```python
from build123d import *

# Parameters (mm, degrees)
SZKIC1_W                    = 140
SZKIC1_H                    = 50
DODANIE_WYCI_GNI_CIE1_DEPTH = 2
DODANIE_WYCI_GNI_CIE2_DEPTH = 12
SFAZOWANIE1_SIZE            = 5


with BuildPart() as part:
    # Szkic1 → Dodanie-wyciągnięcie1 (new body)
    with BuildSketch(Plane.XY):
        Rectangle(SZKIC1_W, SZKIC1_H)
        with BuildLine():
            ThreePointArc((-14.432240892, 12.367994391), (-11.873973335, 6.417701356), (-11, 0))
            ThreePointArc((-11, 0), (-13.243691419, -10.132276987), (-19.555253078, -18.370078729))
            ThreePointArc((-19.555253078, -18.370078729), (-18.936918944, -19.082957273), (-18.714285714, -20))
            ThreePointArc((-18.714285714, -20), (-20.427440625, -21.97932309), (-22.632005609, -20.567759108))
            ThreePointArc((-22.632005609, -20.567759108), (-38.945575695, -23.673454172), (-53.370078729, -15.444746922))
            ThreePointArc((-53.370078729, -15.444746922), (-56.627466942, -15.448190673), (-55.567759108, -12.367994391))
            ThreePointArc((-55.567759108, -12.367994391), (-58.673454172, 3.945575695), (-50.444746922, 18.370078729))
            ThreePointArc((-50.444746922, 18.370078729), (-50.448190673, 21.627466942), (-47.367994391, 20.567759108))
            ThreePointArc((-47.367994391, 20.567759108), (-31.054424305, 23.673454172), (-16.629921271, 15.444746922))
            ThreePointArc((-16.629921271, 15.444746922), (-14.391659035, 16.190949513), (-13, 14.285714286))
            ThreePointArc((-13, 14.285714286), (-13.397577113, 13.088951614), (-14.432240892, 12.367994391))
        make_face(mode=Mode.SUBTRACT)
        with BuildLine():
            ThreePointArc((50.444746922, 18.370078729), (56.756308581, 10.132276987), (59, 0))
            ThreePointArc((59, 0), (58.126026665, -6.417701356), (55.567759108, -12.367994391))
            ThreePointArc((55.567759108, -12.367994391), (56.602422887, -13.088951614), (57, -14.285714286))
            ThreePointArc((57, -14.285714286), (55.608340965, -16.190949513), (53.370078729, -15.444746922))
            ThreePointArc((53.370078729, -15.444746922), (38.945575695, -23.673454172), (22.632005609, -20.567759108))
            ThreePointArc((22.632005609, -20.567759108), (19.551809327, -21.627466942), (19.555253078, -18.370078729))
            ThreePointArc((19.555253078, -18.370078729), (11.326545828, -3.945575695), (14.432240892, 12.367994391))
            ThreePointArc((14.432240892, 12.367994391), (13.372533058, 15.448190673), (16.629921271, 15.444746922))
            ThreePointArc((16.629921271, 15.444746922), (31.054424305, 23.673454172), (47.367994391, 20.567759108))
            ThreePointArc((47.367994391, 20.567759108), (49.572559375, 21.97932309), (51.285714286, 20))
            ThreePointArc((51.285714286, 20), (51.063081056, 19.082957273), (50.444746922, 18.370078729))
        make_face(mode=Mode.SUBTRACT)
    extrude(amount=DODANIE_WYCI_GNI_CIE1_DEPTH)

    # Szkic2 → Dodanie-wyciągnięcie2 (add)
    with BuildSketch(Plane.XY.offset(2)):
        Polygon((70, 25), (70, -19), (82, -19), (82, -13), (72, -13), (72, 27), (-72, 27), (-72, -13), (-82, -13), (-82, -19), (-70, -19), (-70, 25), align=None)
    extrude(amount=-DODANIE_WYCI_GNI_CIE2_DEPTH)

    # Szkic4 → CBORE for M3 Hex Socket Head Cap Screw1 (revolve, cut)
    with BuildSketch(Plane(origin=(-77, -13, -4), x_dir=(0, 0, 1), z_dir=(1, 0, 0))):
        Polygon((0, 0), (0, 8.66137699), (1.6, 7.7), (1.6, 3.4), (3.25, 3.4), (3.25, 0), align=None)
    cbore_for_m3_hex_socket_head_cap_screw1 = revolve(axis=Axis((-77, -6.65, -4), (0, -1, 0)), mode=Mode.SUBTRACT)

    # Lustro1: CBORE for M3 Hex Socket Head Cap Screw1 across plane
    add(cbore_for_m3_hex_socket_head_cap_screw1.mirror(Plane(origin=(0, 0, 0), x_dir=(0, 0, 1), z_dir=(1, 0, 0))), mode=Mode.SUBTRACT)

    # Sfazowanie1
    # the kernel refuses this chamfer: 5 mm, written as the material it takes off along each edge
    with BuildSketch(Plane(origin=(-82, -13, 14.85841494), x_dir=(0.9996219169112968, 0.027495876610586625, 0), z_dir=(0, 0, -1)), Plane(origin=(82, -13, 14.85841494), x_dir=(0.027495876610590466, -0.9996219169112965, 0), z_dir=(0, 0, -1))) as sfazowanie1_piece_1:
        Polygon((SFAZOWANIE1_SIZE * 0.999621916911, SFAZOWANIE1_SIZE * 0.0274958766106), (-SFAZOWANIE1_SIZE * 0.0274958766106, SFAZOWANIE1_SIZE * 0.999621916911), (0, 0), align=None)
    extrude(amount=37.71682988, mode=Mode.SUBTRACT)


solid = part.part
```
CAD build for the part. Positions are in the model's coordinates, mm. A direction names the side the tool comes from. Give positions to 0.01 mm unless a question says otherwise; leave off trailing zeros. Order: outer loops, then holes, each group sorted by start corner. A loop starts at its lowest first (then second) coordinate and runs counter-clockwise, first axis right, second up.
(1) Drill centre lines: L1, parallel to X at y = -18.2, z = -4; L2, parallel to X at y = 8.5, z = 1; L3, parallel to X at y = 13.5, z = 0.5. Where is each one in solid material? Low to high.
(2) Flat gauge pins, fed straight in: pin 1 (2.5 mm diameter, centred on x = 20.71, y = -20, fed in from -Z); pin 2 (4.5 mm diameter, centred on x = -55, y = -14.29, fed in from -Z); pin 3 (3 mm diameter, centred on x = 28, z = -5, fed in from -Y); pin 4 (1 mm diameter, centred on y = -21, z = 1, fed in from +X). Where does each tip first touch, or does it go through?
(3) Saw through at C-C, the plane x = -1. Give the cut face in (y, z).
(4) Mould opens along Z. For faces 1 (the flat face through (75, -19, -4)), 2 (the cylindrical face through (-73.827, -14.676, -4.705)), 3 (the flat face through (0, 26, -10)) say: released by +Z, released by -Z, zero draft, split by the parting line, or undercut.
(5) Saw through at D-D, the plane y = -6. Give the cut face in (x, z).
(6) Saw through at B-B, the plane y = 1.5. Give the cut face in (x, z), then the cut area to 3 significant figures.
(7) Saw through at A-A, the plane z = -4. Give the cut face in (x, y).
(8) Tool access for faces 4 (the cylindrical face through (39.18, -23.633, 0.986)), 5 (the flat face through (72, 7, -4)), 6 (the flat face through (-70, 3, -5)), 7 (the flat face through (-75.6, -16.4, -5.4)): list every direction of +Z, -Z, +X, -X, +Y, -Y with a clear straight run to the whole face (end or side of a thin tool).
Results found:
1. L1: x = -82 to -78.6, -75.4 to -70, 70 to 75.4, 78.6 to 82
1. L2: x = -72 to -57.44, -12.56 to 12.56, 57.44 to 72
1. L3: x = -72 to -54.84, -13.16 to 13.16, 54.84 to 72
2. pin 1: passes through
2. pin 2: stops at z = 0
2. pin 3: stops at y = 25
2. pin 4: stops at x = 70
3. outline: (-25, 0) - (25, 0) - (25, -10) - (27, -10) - (27, 2) - (-25, 2) - close
4. face 1: zero draft
4. face 2: undercut
4. face 3: released by -Z
5. outline: (-72, -10) - (-70, -10) - (-70, 0) - (-58.24, 0) - (-58.24, 2) - (-72, 2) - close; (-11.76, 0) - (11.76, 0) - (11.76, 2) - (-11.76, 2) - close; (58.24, 0) - (70, 0) - (70, -10) - (72, -10) - (72, 2) - (58.24, 2) - close
6. outline: (-72, -10) - (-70, -10) - (-70, 0) - (-58.95, 0) - (-58.95, 2) - (-72, 2) - close; (-11.05, 0) - (11.05, 0) - (11.05, 2) - (-11.05, 2) - close; (58.95, 0) - (70, 0) - (70, -10) - (72, -10) - (72, 2) - (58.95, 2) - close
6. area: 136 mm2
7. outline: (-82, -19) - (-78.6, -19) - (-78.6, -16.4) - (-80.25, -16.4) - (-80.25, -16.25) - (-82, -18) - close; (-75.4, -19) - (-70, -19) - (-70, 25) - (70, 25) - (70, -19) - (75.4, -19) - (75.4, -16.4) - (73.75, -16.4) - (73.75, -13) - (72, -13) - (72, 27) - (-72, 27) - (-72, -13) - (-73.75, -13) - (-73.75, -16.4) - (-75.4, -16.4) - close; (78.6, -19) - (82, -19) - (82, -18) - (80.25, -16.25) - (80.25, -16.4) - (78.6, -16.4) - close
8. face 4: +Z, -Z
8. face 5: +Z, -Z, +X, +Y
8. face 6: -Z, -Y
8. face 7: +Y
